from build123d import *

# Parameters (mm, degrees)
F0_R     = 1.85
F1_DEPTH = 1
F2_DEPTH = 5


with BuildPart() as f1:
    # F0 (on Top) → F1 (new body)
    with BuildSketch(Plane.XY):
        with BuildLine():
            ThreePointArc((4, 0), (2.8284271247, 2.8284271247), (0, 4))
            ThreePointArc((0, 4), (-2.8284271247, 2.8284271247), (-4, 0))
            ThreePointArc((-4, 0), (-2.8284271247, -2.8284271247), (0, -4))
            ThreePointArc((0, -4), (2.8284271247, -2.8284271247), (4, 0))
        make_face()
        Circle(F0_R, mode=Mode.SUBTRACT)
        with BuildLine():
            Line((0, 4), (-4, 4))
            Line((-4, 4), (-4, 0))
            ThreePointArc((-4, 0), (-2.8284271247, 2.8284271247), (0, 4))
        make_face()
        with BuildLine():
            Line((4, 4), (0, 4))
            ThreePointArc((0, 4), (2.8284271247, 2.8284271247), (4, 0))
            Line((4, 0), (4, 4))
        make_face()
        with BuildLine():
            ThreePointArc((0, -4), (-2.8284271247, -2.8284271247), (-4, 0))
            Line((-4, 0), (-4, -4))
            Line((-4, -4), (0, -4))
        make_face()
        with BuildLine():
            Line((4, -4), (4, 0))
            ThreePointArc((4, 0), (2.8284271247, -2.8284271247), (0, -4))
            Line((0, -4), (4, -4))
        make_face()
    extrude(amount=F1_DEPTH)

    # F0 (on Top) → F2 (join)
    with BuildSketch(Plane.XY):
        with BuildLine():
            ThreePointArc((4, 0), (2.8284271247, 2.8284271247), (0, 4))
            ThreePointArc((0, 4), (-2.8284271247, 2.8284271247), (-4, 0))
            ThreePointArc((-4, 0), (-2.8284271247, -2.8284271247), (0, -4))
            ThreePointArc((0, -4), (2.8284271247, -2.8284271247), (4, 0))
        make_face()
        Circle(F0_R, mode=Mode.SUBTRACT)
    extrude(amount=F2_DEPTH)


solid = f1.part
Geometry check sheet. Reference: the model listing, model coordinates, mm. A direction names the side the tool comes from. Round coordinates to 2 decimals unless told otherwise and drop trailing zeros. Order: outer loops, then holes, each group sorted by start corner. A loop starts at its lowest first (then second) coordinate and runs counter-clockwise, first axis right, second up. Notation, with made-up numbers: M -21,27 L 21,27 A24 ccw 21,53 Z; hole C 77.5,40.25 d3. An arc over 180 degrees is marked long. Answer in a Markdown table with one row per item. Add a question column.
Item 1: Sectioned sample at D-D, the plane x = -2.75. Enter the section's corners in (y, z).
Item 2: Sectioned sample at C-C, the plane x = -1.25. Enter the section's corners in (y, z), plus the area to 3 significant figures.
Item 3: Sectioned sample at A-A, the plane z = 1.5. Enter the section's corners in (x, y).
Item 4: Sectioned sample at B-B, the plane y = -1.5. Enter the section's corners in (x, z), plus the area to 3 significant figures.
Item 5: Material ranges on L1, parallel to Y at x = -1.25, z = 2.1; L2, parallel to X at y = -0.5, z = 1.1; L3, parallel to Z at x = 2, y = -3.5, recorded low to high. Write a range as [from, to].
Item 6: Set-up check for faces 4 (the face through (-3, 3, 1)), 5 (the face through (3, -3, 1)), 6 (the face through (3, 3, 1)): record each of +Z, -Z, +X, -X, +Y, -Y from which the full face is reachable in a straight line by a thin tool's end or side.
Item 7: Draft check along Y on faces 1 (the face through (-0.401, -1.806, 2.465)), 2 (the face through (-3, -3, 1)), 3 (the face through (0.1, 4, 0.5)). Enter one of: released by +Y, released by -Y, zero draft, split by the parting line, or undercut.
Filled in:
| question | item | result |
|---|---|---|
| 1 | outline | M -4,0 L 4,0 L 4,1 L 2.9,1 L 2.9,5 L -2.9,5 L -2.9,1 L -4,1 Z |
| 2 | outline | M -4,0 L -1.36,0 L -1.36,5 L -3.8,5 L -3.8,1 L -4,1 Z; M 1.36,0 L 4,0 L 4,1 L 3.8,1 L 3.8,5 L 1.36,5 Z |
| 2 | area | 24.8 mm² |
| 3 | outline | C 0,0 d8; hole C 0,0 d3.7 |
| 4 | outline | M -4,0 L -1.08,0 L -1.08,5 L -3.71,5 L -3.71,1 L -4,1 Z; M 1.08,0 L 4,0 L 4,1 L 3.71,1 L 3.71,5 L 1.08,5 Z |
| 4 | area | 26.8 mm² |
| 5 | L1 | y = [-3.8, -1.36], [1.36, 3.8] |
| 5 | L2 | x = [-3.97, -1.78], [1.78, 3.97] |
| 5 | L3 | z = [0, 1] |
| 6 | face 4 | +Z, -X, +Y |
| 6 | face 5 | +Z, +X, -Y |
| 6 | face 6 | +Z, +X, +Y |
| 7 | face 1 | undercut |
| 7 | face 2 | zero draft |
| 7 | face 3 | released by +Y |
